Part model, mm, in its own coordinate system. Coordinates: 2 decimals unless noted, no trailing zeros. Loops run counter-clockwise (first coordinate to the right, second up) from the corner with the lowest first, then second, coordinate; pieces in that order, holes last. Notation, with made-up numbers: (45.5, 46) -> (63.5, 46) arc R18 ccw to (63.5, 51) -> close; hole circle Ø11 at (-3, 14). An arc over 180 degrees is marked (long way). One line per item, written item: value. Start each with the question number.
from build123d import *

# Parameters (mm, degrees)
BOSS_EXTRUDE1_DEPTH = 3.175
FILLET1_R           = 0.79375
FILLET2_R           = 1.5875


# Read off the part's stored shape, not the designer's step: Boss-Extrude1
with BuildPart() as part:
    # Boss-Extrude1 outline → Boss-Extrude1 (new body)
    with BuildSketch(Plane.XY):
        with BuildLine():
            ThreePointArc((252.73, 90.4494), (265.43, 103.1494), (252.73, 115.8494))
            Line((252.73, 115.8494), (252.73, 206.2988))
            Line((252.73, 206.2988), (0, 206.2988))
            Line((0, 206.2988), (0, 0))
            Line((0, 0), (252.73, 0))
            Line((252.73, 0), (252.73, 90.4494))
        make_face()
    extrude(amount=BOSS_EXTRUDE1_DEPTH)

    # Fillet1
    fillet1_edges = [part.edges().sort_by_distance(p)[0] for p in [
        (252.73, 0, 1.5875),
        (0, 0, 1.5875),
        (0, 206.2988, 1.5875),
        (252.73, 206.2988, 1.5875),
    ]]
    fillet(fillet1_edges, radius=FILLET1_R)

    # Fillet2
    fillet2_edges = [part.edges().sort_by_distance(p)[0] for p in [
        (252.73, 90.4494, 1.5875),
        (252.73, 115.8494, 1.5875),
    ]]
    fillet(fillet2_edges, radius=FILLET2_R)


solid = part.part
1) Probe line 1 (X direction, y = 88, z = 1.4); line 2 (X direction, y = 105, z = 1.2). List the from-to ranges inside material, lowest first. Write a range as from..to.
2) Slice it at A-A (z = 0.65). Give the cut face in (x, y) (1 decimal), then the cut area to 3 significant figures.
3) Slice it at B-B (y = 40.5). Give the cut face in (x, z) (3 decimals).
Check sheet entries:
1. line 1: x = 0..252.73
1. line 2: x = 0..265.29
2. outline: (0, 0.8) arc R0.8 ccw to (0.8, 0) -> (251.9, 0) arc R0.8 ccw to (252.7, 0.8) -> (252.7, 89) arc R1.6 cw to (254.1, 90.5) arc R12.7 ccw to (254.1, 115.8) arc R1.6 cw to (252.7, 117.3) -> (252.7, 205.5) arc R0.8 ccw to (251.9, 206.3) -> (0.8, 206.3) arc R0.8 ccw to (0, 205.5) -> close
2. area: 52,400 mm^2
3. outline: (0, 0) -> (252.73, 0) -> (252.73, 3.175) -> (0, 3.175) -> close
